```python
from build123d import *

# Parameters (mm, degrees)
F1_DEPTH = 10.922
F2_DEPTH = 60.198
F0_W     = 12.6999963462
F0_H     = 22.8600017996
F3_DEPTH = 50.8
F5_DEPTH = 25.4
F6_R     = 9.525
F7_DEPTH = 25.4
F8_DEPTH = 25.4


with BuildPart() as f1:
    # F0 (on Front) → F1 (new body)
    with BuildSketch(Plane.XZ):
        Polygon((10.2849198341, 23.9218054244), (-13.2440533489, 23.9218054244), (-40.5150838196, 23.9218054244), (-40.5150838196, 1.0618036248), align=None)
    extrude(amount=F1_DEPTH)

    # F0 (on Front) → F2 (join)
    with BuildSketch(Plane.XZ):
        Polygon((-13.2440533489, 39.1618055656), (-53.2150801659, 39.1618055656), (-53.2150801659, 23.9218054244), (-40.5150838196, 23.9218054244), (-13.2440533489, 23.9218054244), align=None)
        Polygon((61.0849198341, 39.1618055656), (-13.2440533489, 39.1618055656), (-13.2440533489, 23.9218054244), (10.2849198341, 23.9218054244), (61.0849198341, 23.9218054244), align=None)
    extrude(amount=F2_DEPTH)

    # F0 (on Front) → F3 (join)
    with BuildSketch(Plane.XZ):
        with Locations((-46.8650819927, 12.4918045246)):
            Rectangle(F0_W, F0_H)
    extrude(amount=F3_DEPTH)

    # F4 (on face) → F5 (cut)
    with BuildSketch(Plane.YZ.offset(-40.5150838196)):
        Polygon((-23.4362483025, 1.0618036248), (-50.8, 12.4918045246), (-50.8, 1.0618036248), align=None)
    extrude(amount=-F5_DEPTH, mode=Mode.SUBTRACT)

    # F6 (on face) → F7 (cut)
    with BuildSketch(Plane(origin=(0, 0, 23.9218054244), x_dir=(1, 0, 0), z_dir=(0, 0, -1))):
        Polygon((61.0849198341, 60.198), (-27.1072126925, 60.198), (61.0849198341, 45.0329519808), align=None)
        with Locations((40.7223813236, 23.666460067)):
            Circle(F6_R)
    extrude(amount=-F7_DEPTH, mode=Mode.SUBTRACT)

    # F6 (on face) → F8 (cut)
    with BuildSketch(Plane(origin=(0, 0, 23.9218054244), x_dir=(1, 0, 0), z_dir=(0, 0, -1))):
        Polygon((61.0849198341, 60.198), (-27.1072126925, 60.198), (61.0849198341, 45.0329519808), align=None)
        with Locations((40.7223813236, 23.666460067)):
            Circle(F6_R)
    extrude(amount=-F8_DEPTH, mode=Mode.SUBTRACT)


solid = f1.part
```
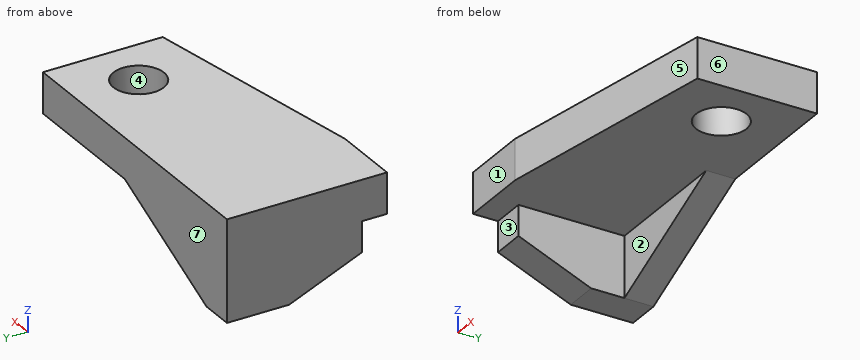
CAD build for the part. Positions are in the model's coordinates, mm. Face numbers are marked on the shaded views. A direction names the side the tool comes from. Round coordinates to 2 decimals unless told otherwise and drop trailing zeros. Order: outer loops, then holes, each group sorted by start corner. A loop starts at its lowest first (then second) coordinate and runs counter-clockwise, first axis right, second up.
Item 1: Probe line 1 along X through (y, z) = (-43, 19.5); line 2 along Z through (x, y) = (42.5, -12); line 3 along Y through (x, z) = (-19.5, 21). List the from-to ranges inside material, lowest first.
Item 2: Tool access for the marked faces 1, 2 and 3: list every direction of +Z, -Z, +X, -X, +Y, -Y with a clear straight run to the whole face (end or side of a thin tool).
Item 3: Mould opens along Y. For the marked faces 4, 5, 6 and 7 say: pulls with the +Y half, pulls with the -Y half, needs draft (parallel to the pull), parting line crosses it, or undercut.
Item 4: Saw through at B-B on y = -5.5. Write the cut outline in (x, z).
Item 5: Saw through at A-A on x = 34. Write the cut outline in (y, z).
Item 6: Saw through at D-D on z = 35. Write the cut outline in (x, y) (3 decimals).
Item 7: Pin check, flat tips, straight feed: pin 1 (9 mm diameter, centred on x = -44, z = 16, fed in from -Y); pin 2 (12 mm diameter, centred on x = 40, y = -47, fed in from -Z); pin 3 (2 mm diameter, centred on x = -5, z = 32, fed in from +Y); pin 4 (11.5 mm diameter, centred on x = -26, z = 14.5, fed in from -Y). Stop position of each tip, or through.
Item 8: Saw through at C-C on z = 10. Write the cut outline in (x, y).
Reported:
1. line 1: x = -53.22 to -40.52
1. line 2: z = 23.92 to 39.16
1. line 3: y = -10.92 to 0
2. face 1: +Z, -Z, +X, -X, -Y
2. face 2: -Z, +X, -Y
2. face 3: -Z, +X, -X, -Y
3. face 4: undercut
3. face 5: pulls with the -Y half
3. face 6: needs draft
3. face 7: pulls with the +Y half
4. outline: (-53.22, 1.06) - (-40.52, 1.06) - (10.28, 23.92) - (61.08, 23.92) - (61.08, 39.16) - (-53.22, 39.16) - close
5. outline: (-49.69, 23.92) - (-30.41, 23.92) - (-30.41, 39.16) - (-49.69, 39.16) - close; (-16.92, 23.92) - (0, 23.92) - (0, 39.16) - (-16.92, 39.16) - close
6. outline: (-53.215, -60.198) - (-27.107, -60.198) - (61.085, -45.033) - (61.085, 0) - (-53.215, 0) - close; hole circle Ø19.05 at (40.722, -23.666)
7. pin 1: stops at y = -50.8
7. pin 2: stops at z = 23.92
7. pin 3: stops at y = 0
7. pin 4: stops at y = -10.92
8. outline: (-53.22, -44.83) - (-40.52, -44.83) - (-40.52, -10.92) - (-20.65, -10.92) - (-20.65, 0) - (-53.22, 0) - close
